from build123d import *

# Parameters (mm, degrees)
SKETCH_1_R                           = 21
EXTRUDE_1_DEPTH                      = 66.5
SKETCH_2_R                           = 13
EXTRUDE_2_DEPTH                      = 2
SKETCH_3_R                           = 5
EXTRUDE_3_DEPTH                      = 24
CUT_EXTRUDE_1_DEPTH                  = 98.1506562
CUT_EXTRUDE_1_DEPTH_BACK             = 19.5
CHAMFER_1_SIZE                       = 0.5
PATTERN_CIRCULAR_1_COUNT             = 4
CHAMFER_1_OF_PATTERN_CIRCULAR_1_SIZE = 0.5
SKETCH_30_R                          = 3.5
EXTRUDE_4_DEPTH                      = 5
SKETCH_31_R                          = 8.25
EXTRUDE_5_DEPTH                      = 1
CUT_EXTRUDE_4_DEPTH                  = 5
CUT_EXTRUDE_START                    = -1
SKETCH_38_R                          = 21
SKETCH_38_R_2                        = 20.5
CUT_EXTRUDE_8_DEPTH                  = 1
EXTRUDE_8_DEPTH                      = 5
EXTRUDE_9_DEPTH                      = 5
SKETCH_37_W                          = 2.259014744
SKETCH_37_H                          = 4.906548019
EXTRUDE_10_DEPTH                     = 6
EXTRUDE_10_TAPER                     = 3
SKETCH_39_R                          = 21
SKETCH_39_R_2                        = 20.5
CUT_EXTRUDE_9_DEPTH                  = 0.5
SKETCH_41_R                          = 21
SKETCH_41_R_2                        = 20.5
CUT_EXTRUDE_10_DEPTH                 = 1
SKETCH_42_R                          = 21
SKETCH_42_R_2                        = 20.5
CUT_EXTRUDE_11_DEPTH                 = 1
CUT_EXTRUDE_12_REACH                 = 95.761
PATTERN_CIRCULAR_4_COUNT             = 12
CUT_EXTRUDE_13_REACH                 = 79.917
PATTERN_CIRCULAR_5_COUNT             = 12
HOLE_WIZARD_M3_1_D                   = 2.5
HOLE_WIZARD_M3_1_DEPTH               = 6
HOLE_WIZARD_M3_1_TIP                 = 0.751075774
SKETCH_13_R                          = 3
CUT_EXTRUDE_14_DEPTH                 = 3
CUT_EXTRUDE_15_DEPTH                 = 1


with BuildPart() as part:
    # 草图1 → 凸台-拉伸1 (new body)
    with BuildSketch(Plane.XY):
        Circle(SKETCH_1_R)
    extrude(amount=EXTRUDE_1_DEPTH)

    # 草图2 → 凸台-拉伸2 (add)
    with BuildSketch(Plane(origin=(0, 0, 0), x_dir=(-1, 0, 0), z_dir=(0, 0, -1))):
        with Locations(Location((0, 0, 0), (0, 0, 180))):
            Circle(SKETCH_2_R)
    extrude(amount=EXTRUDE_2_DEPTH)

    # 草图3 → 凸台-拉伸3 (add)
    with BuildSketch(Plane(origin=(0, 0, -2), x_dir=(-1, 0, 0), z_dir=(0, 0, -1))):
        Circle(SKETCH_3_R)
    extrude(amount=EXTRUDE_3_DEPTH)

    # 草图4 → 切除-拉伸1 (cut, two sides: drawn at the far end of the back side and taken through both)
    with BuildSketch(Plane(origin=(0, 0, -26), x_dir=(-1, 0, 0), z_dir=(0, 0, -1)).offset(-CUT_EXTRUDE_1_DEPTH_BACK)):
        Polygon((54.209292642, -59.866146891), (-0.707106781, -4.949747468), (-4.949747468, -0.707106781), (-59.866146891, 54.209292642), (-169.698945737, -55.623506204), (-55.623506204, -169.698945737), align=None)
    extrude(amount=CUT_EXTRUDE_1_DEPTH + CUT_EXTRUDE_1_DEPTH_BACK, mode=Mode.SUBTRACT)

    # 草图12 → #8-36 螺纹孔1 (revolve, cut)
    with BuildSketch(Plane(origin=(0, 17.5, 0), x_dir=(0, 1, 0), z_dir=(1, 0, 0))):
        Polygon((0, 0), (0, 11.6517212), (1.999999937, 10.45), (1.999999937, 0), align=None)
    hole_wizard_8_36_1 = revolve(axis=Axis((0, 17.5, -6.35), (0, 0, 1)), mode=Mode.SUBTRACT)

    # 倒角1
    chamfer_1_edges = [part.edges().sort_by_distance(p)[0] for p in [
        (0, 15.500000063, 0),
    ]]
    chamfer(chamfer_1_edges, length=CHAMFER_1_SIZE)

    # 阵列(圆周)1: #8-36 螺纹孔1 ×4 about axis
    pattern_circular_1_axis = Axis((0, 0, 0), (0, 0, 1))
    for i in range(1, PATTERN_CIRCULAR_1_COUNT):
        add(hole_wizard_8_36_1.rotate(pattern_circular_1_axis, i * 360 / PATTERN_CIRCULAR_1_COUNT), mode=Mode.SUBTRACT)

    # 倒角1 of 阵列(圆周)1
    chamfer_1_of_pattern_circular_1_edges = [part.edges().sort_by_distance(p)[0] for p in [
        (-15.500000063, 0, 0),
        (0, -15.500000063, 0),
        (15.500000063, 0, 0),
    ]]
    chamfer(chamfer_1_of_pattern_circular_1_edges, length=CHAMFER_1_OF_PATTERN_CIRCULAR_1_SIZE)

    # 草图30 → 凸台-拉伸4 (add)
    with BuildSketch(Plane.XY.offset(66.5)):
        Circle(SKETCH_30_R)
    extrude(amount=EXTRUDE_4_DEPTH)

    # 草图31 → 凸台-拉伸5 (add)
    with BuildSketch(Plane(origin=(0, 0, -2), x_dir=(-1, 0, 0), z_dir=(0, 0, -1))):
        Circle(SKETCH_31_R)
    extrude(amount=EXTRUDE_5_DEPTH)

    # Sketch 3D_5 → 切除-拉伸4 (cut)
    with BuildSketch(Plane(origin=(21.698598574, 0, 41.5), x_dir=(-0.8701153178040487, -0.49284818526881014, 0), z_dir=(0, 0, -1))):
        with BuildLine():
            Line((0, 0), (2.265924322, 8.186168064))
            Line((2.265924322, 8.186168064), (31.840322246, 0))
            Line((31.840322246, 0), (29.574397924, -8.186168064))
            ThreePointArc((29.574397924, -8.186168064), (13.091788044, -10.218142392), (0, 0))
        make_face()
    extrude(amount=-CUT_EXTRUDE_4_DEPTH, mode=Mode.SUBTRACT)

    # 草图38 → 切除-拉伸8 (cut)
    with BuildSketch(Plane.XY.offset(48.5).offset(CUT_EXTRUDE_START)):
        Circle(SKETCH_38_R)
        Circle(SKETCH_38_R_2, mode=Mode.SUBTRACT)
    extrude(amount=CUT_EXTRUDE_8_DEPTH, mode=Mode.SUBTRACT)

    # 草图35 → 凸台-拉伸8 (add)
    with BuildSketch(Plane(origin=(0, 0, 46.5), x_dir=(-1, 0, 0), z_dir=(0, 0, -1))):
        Polygon((-19.650844704, 0.722539425), (-13.558326759, -7.216544928), (-10.385037772, -4.781337133), (-16.604585732, 3.323278452), (-19.650844704, 0.985554524), align=None)
    extrude(amount=EXTRUDE_8_DEPTH)

    # 草图36 → 凸台-拉伸9 (add)
    with BuildSketch(Plane(origin=(0, 0, 46.5), x_dir=(-1, 0, 0), z_dir=(0, 0, -1))):
        Polygon((0, -18.923068099), (-7.58749284, -12.409240314), (-4.981961726, -9.374243178), (2.605531114, -15.888070963), align=None)
    extrude(amount=EXTRUDE_9_DEPTH)

    # 草图37 → 凸台-拉伸10 (add)
    with BuildSketch(Plane(origin=(12.018490008, -9.223087045, 0), x_dir=(0, 0, -1), z_dir=(0.793322246809358, -0.6088019486806462, 0))):
        with Locations((-44.496547362, 7.679113422)):
            Rectangle(SKETCH_37_W, SKETCH_37_H)
    extrude(amount=EXTRUDE_10_DEPTH, taper=EXTRUDE_10_TAPER)

    # 草图39 → 切除-拉伸9 (cut)
    with BuildSketch(Plane(origin=(0, 0, 36), x_dir=(-1, 0, 0), z_dir=(0, 0, -1))):
        Circle(SKETCH_39_R)
        with Locations(Location((0, 0, 0), (0, 0, 180))):
            Circle(SKETCH_39_R_2, mode=Mode.SUBTRACT)
    extrude(amount=-CUT_EXTRUDE_9_DEPTH, mode=Mode.SUBTRACT)

    # 草图41 → 切除-拉伸10 (cut)
    with BuildSketch(Plane(origin=(0, 0, 38), x_dir=(-1, 0, 0), z_dir=(0, 0, -1))):
        Circle(SKETCH_41_R)
        Circle(SKETCH_41_R_2, mode=Mode.SUBTRACT)
    extrude(amount=-CUT_EXTRUDE_10_DEPTH, mode=Mode.SUBTRACT)

    # 草图42 → 切除-拉伸11 (cut)
    with BuildSketch(Plane(origin=(0, 0, 40), x_dir=(-1, 0, 0), z_dir=(0, 0, -1))):
        Circle(SKETCH_42_R)
        Circle(SKETCH_42_R_2, mode=Mode.SUBTRACT)
    extrude(amount=-CUT_EXTRUDE_11_DEPTH, mode=Mode.SUBTRACT)

    # 草图43 → 切除-拉伸12 (cut, up to next)
    with BuildSketch(Plane.XY.offset(62.5), mode=Mode.PRIVATE) as cut_extrude_12_sk1:
        with BuildLine():
            Line((0, 18.5), (0, 21))
            ThreePointArc((0, 21), (-3.864852633, 20.641291484), (-7.597671404, 19.577420393))
            Line((-7.597671404, 19.577420393), (-6.693186713, 17.246775108))
            ThreePointArc((-6.693186713, 17.246775108), (-3.404751129, 18.183994879), (0, 18.5))
        make_face()
    cut_extrude_12_tool1 = extrude(cut_extrude_12_sk1.sketch, amount=CUT_EXTRUDE_12_REACH, mode=Mode.PRIVATE) & part.part
    cut_extrude_12 = cut_extrude_12_tool1.solids().sort_by_distance((-3.618908, 19.327758, 62.5))[0]
    add(cut_extrude_12, mode=Mode.SUBTRACT)

    # 阵列(圆周)4: 切除-拉伸12 ×12 about axis
    pattern_circular_4_axis = Axis((0, 0, 0), (0, 0, 1))
    for i in range(1, PATTERN_CIRCULAR_4_COUNT):
        add(cut_extrude_12.rotate(pattern_circular_4_axis, i * 360 / PATTERN_CIRCULAR_4_COUNT), mode=Mode.SUBTRACT)

    # 切除-拉伸13: up to this plane
    cut_extrude_13_end = Plane(origin=(-6.693186713, 17.246775108, 71.501), z_dir=(0.9322581139355903, 0.36179387640099137, 0))
    # 草图45 → 切除-拉伸13 (cut, up to the surface)
    with BuildSketch(Plane(origin=(0, 0, 0), x_dir=(0, 0, 1), z_dir=(-0.8660254037844382, -0.5000000000000011, 0)), mode=Mode.PRIVATE) as cut_extrude_13_sk1:
        Polygon((62.5, 21), (66.5, 18.5), (66.5, 21), align=None)
    cut_extrude_13_tool1 = split(extrude(cut_extrude_13_sk1.sketch, amount=-CUT_EXTRUDE_13_REACH, mode=Mode.PRIVATE), bisect_by=cut_extrude_13_end, keep=Keep.BOTH, mode=Mode.PRIVATE)
    cut_extrude_13 = cut_extrude_13_tool1.solids().sort_by_distance((-10.083333, 17.464846, 65.166667))[0]
    add(cut_extrude_13, mode=Mode.SUBTRACT)

    # 阵列(圆周)5: 切除-拉伸13 ×12 about axis
    pattern_circular_5_axis = Axis((0, 0, 0), (0, 0, 1))
    for i in range(1, PATTERN_CIRCULAR_5_COUNT):
        add(cut_extrude_13.rotate(pattern_circular_5_axis, i * 360 / PATTERN_CIRCULAR_5_COUNT), mode=Mode.SUBTRACT)

    # M3 螺纹孔1
    with Locations(Plane.XY.offset(66.5)):
        with Locations((-6.5, 0), (6.5, 0)):
            Hole(HOLE_WIZARD_M3_1_D / 2, depth=HOLE_WIZARD_M3_1_DEPTH)
            with Locations((0, 0, -(HOLE_WIZARD_M3_1_DEPTH + HOLE_WIZARD_M3_1_TIP / 2))):  # 118° drill point
                Cone(0, HOLE_WIZARD_M3_1_D / 2, HOLE_WIZARD_M3_1_TIP, mode=Mode.SUBTRACT)

    # 草图13 → 切除-拉伸14 (cut)
    with BuildSketch(Plane(origin=(0, 0, 0), x_dir=(-1, 0, 0), z_dir=(0, 0, -1))):
        with Locations((12.374368671, -12.374368671)):
            Circle(SKETCH_13_R)
        with Locations(Location((12.374368671, 12.374368671, 0), (0, 0, 180))):
            Circle(SKETCH_13_R)
        with Locations(Location((-12.374368671, -12.374368671, 0), (0, 0, 180))):
            Circle(SKETCH_13_R)
        with Locations((-12.374368671, 12.374368671)):
            Circle(SKETCH_13_R)
    extrude(amount=-CUT_EXTRUDE_14_DEPTH, mode=Mode.SUBTRACT)

    # 草图52 → 切除-拉伸15 (cut)
    with BuildSketch(Plane(origin=(0, 0, 3), x_dir=(-1, 0, 0), z_dir=(0, 0, -1))):
        Polygon((13.817744344, 12.374368671), (13.096056507, 13.624368671), (11.652680834, 13.624368671), (10.930992998, 12.374368671), (11.652680834, 11.124368671), (13.096056507, 11.124368671), align=None)
        Polygon((-13.096056507, 11.124368671), (-13.817744344, 12.374368671), (-13.096056507, 13.624368671), (-11.652680834, 13.624368671), (-10.930992998, 12.374368671), (-11.652680834, 11.124368671), align=None)
        Polygon((-13.817744344, -12.374368671), (-13.096056507, -13.624368671), (-11.652680834, -13.624368671), (-10.930992998, -12.374368671), (-11.652680834, -11.124368671), (-13.096056507, -11.124368671), align=None)
        Polygon((13.096056507, -11.124368671), (13.817744344, -12.374368671), (13.096056507, -13.624368671), (11.652680834, -13.624368671), (10.930992998, -12.374368671), (11.652680834, -11.124368671), align=None)
    extrude(amount=-CUT_EXTRUDE_15_DEPTH, mode=Mode.SUBTRACT)


solid = part.part
CAD build for the part. Positions are in the model's coordinates, mm. A direction names the side the tool comes from. Round coordinates to 2 decimals unless told otherwise and drop trailing zeros. Write each loop counter-clockwise with the first axis right and the second up, starting at its lowest first coordinate (ties: lowest second). Pieces come first, ordered by that corner, then holes.
(1) Probe line 1 along X through (y, z) = (-0.5, 8.5); line 2 along Z through (x, y) = (1, -10.5); line 3 along Z through (x, y) = (-10, 9.5). List the from-to ranges inside material, lowest first.
(2) Slice it at B-B, the plane z = 21. Write the cut outline in (x, y), and give its area (3 significant figures).
(3) 3-axis set-ups, long thin cutter, end or side, ignore diameter. For faces 5 (the face through (-16.33, 11.25, 64.47)), 6 (the face through (-7.62, -3.16, -2.49)), 7 (the face through (13.45, -0.79, 44.04)): which of +Z, -Z, +X, -X, +Y, -Y reach the whole face in a straight line?
(4) Mould opens along Y. For faces 1 (the face through (-18.175, -3.452, 64.472)), 2 (the face through (20.03, 6.31, 39.49)), 3 (the face through (-18.6, -9.2, 36)), 4 (the face through (-2.98, -19.26, 64.03)) say: pulls with the +Y half, pulls with the -Y half, needs draft (parallel to the pull), parting line crosses it, or undercut.
(5) Drop flat-ended pins along their axis: P1, Ø5, axis at y = 9.5, z = 2, coming from the -X side; P2, Ø8, axis at x = 4.5, y = -10.5, coming from the +Z side; P3, Ø0.5, axis at x = -12, z = 3.5, coming from the +Y side; P4, Ø18.5, axis at x = -0.5, y = 6.5, coming from the +Z side. Give the stop position or say it passes through.
(6) Slice it at A-A, the plane z = 7. Write the cut outline in (x, y).
From the geometry:
1. line 1: x = -20.99 to -19.44, -15.56 to 15.56, 19.44 to 20.99
1. line 2: z = -2 to 41.5, 46.5 to 66.5
1. line 3: z = 0 to 66.5
2. outline: circle Ø42 at (0, 0)
2. area: 1,390 mm2
3. face 5: +Z, -X, +Y
3. face 6: -Z
3. face 7: none
4. face 1: undercut
4. face 2: parting line crosses it
4. face 3: needs draft
4. face 4: undercut
5. P1: stops at x = -19.8
5. P2: stops at z = 66.5
5. P3: stops at y = 17.41
5. P4: stops at z = 71.5
6. outline: circle Ø42 at (0, 0); hole circle Ø4 at (-17.5, 0); hole circle Ø4 at (0, -17.5); hole circle Ø4 at (0, 17.5); hole circle Ø4 at (17.5, 0)
